Read the model definition and answer for the solid it produces. Units are mm, in the model's axes. Coordinates: 2 decimals unless noted, no trailing zeros. Write each loop counter-clockwise with the first axis right and the second up, starting at its lowest first coordinate (ties: lowest second). Pieces come first, ordered by that corner, then holes. Notation, with made-up numbers: (30, 19.25) -> (54, 19.25) arc R19 cw to (54, 48.25) -> close; hole circle Ø4 at (78.5, 82.5). An arc over 180 degrees is marked (long way). Write item = value, one per line. Start each with the question number.
1) Section A-A (z = 56) is taken. Determine the outline of the cut face in (x, y), plus the area to 3 significant figures.
2) Find the intervals of material crossed by line 1 along Y through (x, z) = (337.5, 56.75); line 2 along Z through (x, y) = (889.5, -49.25); line 3 along Y through (x, z) = (266.7, 62.4), in increasing order. Write a range as from..to.
3) Flat-ended cylindrical pins translate along their axes: pin 1 Ø10 at (y, z) = (-54, 44) entering from +X; pin 2 Ø7 at (x, y) = (107.95, -47.31) entering from +Z. Find the tip coordinate at first contact, or state that the pin passes through.
4) Section B-B (x = 140.5) is taken. Determine the outline of the cut face in (y, z), plus the area to 3 significant figures.
from build123d import *

# Parameters (mm, degrees)
F0_W     = 25.4
F0_H     = 25.4
F1_DEPTH = 952.5
F2_W     = 19.05
F2_H     = 19.05
F3_DEPTH = 952.501
F5_D     = 7.9375
F5_DEPTH = 17.4752
F5_TIP   = 2.3846655818


with BuildPart() as f1:
    # F0 (on Right) → F1 (new body)
    with BuildSketch(Plane.YZ):
        with Locations((-47.3075013936, 50.5391221166)):
            Rectangle(F0_W, F0_H)
    extrude(amount=F1_DEPTH)

    # F2 (on face) → F3 (cut, through all)
    with BuildSketch(Plane.YZ.offset(952.5)):
        with Locations((-47.3075013936, 50.5391221166)):
            Rectangle(F2_W, F2_H)
    extrude(amount=-F3_DEPTH, mode=Mode.SUBTRACT)

    # F5
    with Locations(Plane.XY.offset(63.2391221166)):
        with Locations((844.55, -47.3075013936), (685.8, -47.3075013936), (476.25, -47.3075013936), (266.7, -47.3075013936), (107.95, -47.3075013936)):
            Hole(F5_D / 2, depth=F5_DEPTH)
            with Locations((0, 0, -(F5_DEPTH + F5_TIP / 2))):  # 118° drill point
                Cone(0, F5_D / 2, F5_TIP, mode=Mode.SUBTRACT)


solid = f1.part
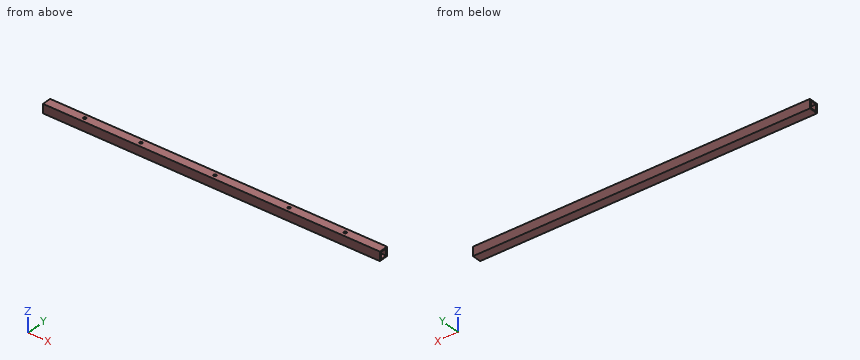
Answer key:
q1.outline = (0, -60.01) -> (952.5, -60.01) -> (952.5, -56.83) -> (0, -56.83) -> close; (0, -37.78) -> (952.5, -37.78) -> (952.5, -34.61) -> (0, -34.61) -> close
q1.area = 6,050 mm^2
q2.line_1 = -60.01..-56.83, -37.78..-34.61
q2.line_2 = 37.84..41.01, 60.06..63.24
q2.line_3 = -60.01..-51.28, -43.34..-34.61
q3.pin_1 = 952.5
q3.pin_2 = 41.01
q4.outline = (-60.01, 37.84) -> (-34.61, 37.84) -> (-34.61, 63.24) -> (-60.01, 63.24) -> close; hole (-56.83, 41.01) -> (-37.78, 41.01) -> (-37.78, 60.06) -> (-56.83, 60.06) -> close
q4.area = 282 mm^2
